Part model, mm, in its own coordinate system. Give positions to 0.01 mm unless a question says otherwise; leave off trailing zeros. Write each loop counter-clockwise with the first axis right and the second up, starting at its lowest first coordinate (ties: lowest second). Pieces come first, ordered by that corner, then holes. Notation, with made-up numbers: M 77.25,-19 L 116.25,-19 A20 ccw 116.25,20 Z; hole C 39,82.25 d2. An arc over 180 degrees is marked long. Answer as CSV lines item,"result". Start each with the question number.
1) Slice it at A-A, the plane y = -63.5. Give the cut face in (x, z), plus the area to 3 significant figures.
2) Pin check, flat tip, straight feed: pin 1 Ø15.5 at (x, y) = (-84, 0) entering from +Z. Stop position of the tip, or through.
3) Slice it at D-D, the plane z = 1.75. Give the number of separate pieces and of enclosed holes in the cut face, plus the area to 3 significant figures.
4) Slice it at B-B, the plane x = 28. Give the cut face in (y, z).
5) Wall check: line 1 along Y through (x, z) = (-28, 4); line 2 along X through (y, z) = (0, 6); line 3 along Y through (x, z) = (84, 2.75). Give the ranges that are in metal, low to high. Write a range as from..to.
6) Slice it at C-C, the plane y = -127. Give the cut face in (x, z).
Autodesk Inventor part; units mm, degrees
ref_plane "YZ Plane" through (0, 0, 0) normal (1, 0, 0) x (0, 1, 0)
ref_plane "XZ Plane" through (0, 0, 0) normal (0, 1, 0) x (-1, 0, 0)
ref_plane "XY Plane" through (0, 0, 0) normal (0, 0, 1) x (1, 0, 0)
sketch "Sketch2" plane through (0, 0, 0) normal (0, 0, 1) x (1, 0, 0)
  line L0 (-53, -96) -> (53, -96)
  line L1 (53, -96) -> (53, 96)
  line L2 (53, 96) -> (-53, 96)
  line L3 (-53, 96) -> (-53, -96)
  line L4 (-53, -96) -> (53, 96) construction
  line L5 (53, -96) -> (-53, 96) construction
  line L6 (-103, -146) -> (103, -146)
  line L7 (103, -146) -> (103, 146)
  line L8 (103, 146) -> (-103, 146)
  line L9 (-103, 146) -> (-103, -146)
  point P0 (0, 0)
  dimension "d29" = 106
  dimension "d30" = 192
  dimension "d31" = 50
extrude "Plate2" add sketch "Sketch2" along normal blind 8
sketch "Sketch5" plane through (0, 0, 8) normal (0, 0, 1) x (1, 0, 0)
  line L0 (53, 96) -> (53, -96) construction
  line L1 (53, -96) -> (-53, -96) construction
  line L2 (-53, -96) -> (-53, 96) construction
  line L3 (-53, 96) -> (53, 96) construction
  line L4 (103, -146) -> (-103, -146) construction
  line L5 (103, 146) -> (103, -146) construction
  line L6 (-103, 146) -> (103, 146) construction
  line L7 (-103, -146) -> (-103, 146) construction
  line L8 (-84, 127) -> (84, 127) construction
  line L9 (84, 127) -> (84, -127) construction
  line L10 (84, -127) -> (-84, -127) construction
  line L11 (-84, -127) -> (-84, 127) construction
  line L12 (-53, 0) -> (53, 0) construction
  line L13 (0, 96) -> (0, -96)
  point P0 (0, 0)
  point P1 (0, -127)
  point P2 (-84, 63.5)
  point P3 (-84, 0)
  point P4 (-84, -63.5)
  point P5 (-28, -127)
  point P6 (28, -127)
  point P7 (84, -63.5)
  point P8 (84, 0)
  point P9 (84, 63.5)
  point P10 (28, 127)
  point P11 (-28, 127)
  dimension "d34" = 19
  dimension "d49" = 63.5
  dimension "d50" = 63.5
  dimension "d51" = 56
  dimension "d52" = 56
  dimension "d53" = 56
fillet "Corner Round1" radius 6 8 edges at (-103, -146, 4) (-103, 146, 4) (103, 146, 4) (103, -146, 4) (53, -96, 4) (-53, -96, 4) (-53, 96, 4) (53, 96, 4)
hole "Hole1" at (-84, 127, 8) at (-84, 63.5, 8) at (-84, 0, 8) at (-84, -63.5, 8) at (-84, -127, 8) at (-28, -127, 8) at (28, -127, 8) at (84, -127, 8) at (84, -63.5, 8) at (84, 0, 8) at (84, 63.5, 8) at (84, 127, 8) at (28, 127, 8) at (-28, 127, 8) direction (0, 0, -1) diameter 17 end through all
equation "\"d29\" = ChargingHatch_hight - 2 * Thickness"
equation "\"d30\" = ChargingHatch_width - 2 * Thickness"
equation "\"d59\" = Thickness"
equation "\"d14\" = Thickness"
equation "\"BendReliefWidth\" = Thickness"
equation "\"BendReliefDepth\" = 0.5 * Thickness"
equation "\"CornerReliefSize\" = 4 * Thickness"
equation "\"MinimumRemnant\" = 2 * Thickness"
equation "\"TransitionRadius\" = BendRadius"
equation "\"JacobiRadiusSize\" = BendRadius"
equation "\"GapSize\" = Thickness"
properties part number "PRS 9606 charging flange round_D1200 940" material "Steel"
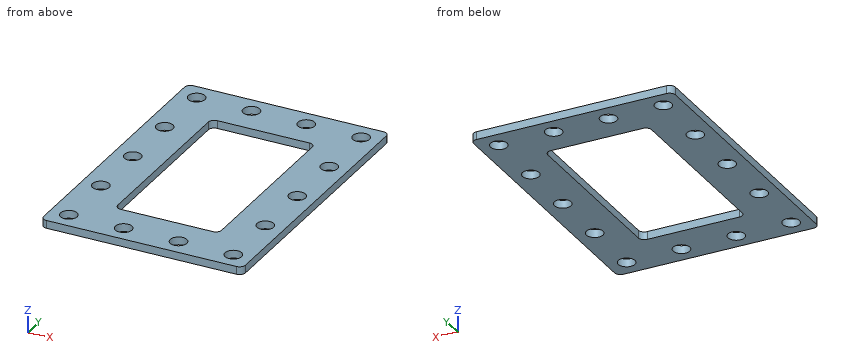
Found:
1,outline,"M -103,0 L -92.5,0 L -92.5,8 L -103,8 Z; M -75.5,0 L -53,0 L -53,8 L -75.5,8 Z; M 53,0 L 75.5,0 L 75.5,8 L 53,8 Z; M 92.5,0 L 103,0 L 103,8 L 92.5,8 Z"
1,area,"528 mm²"
2,pin 1,"through"
3,separate pieces,"1"
3,enclosed holes,"15"
3,area,"36,600 mm²"
4,outline,"M -146,0 L -135.5,0 L -135.5,8 L -146,8 Z; M -118.5,0 L -96,0 L -96,8 L -118.5,8 Z; M 96,0 L 118.5,0 L 118.5,8 L 96,8 Z; M 135.5,0 L 146,0 L 146,8 L 135.5,8 Z"
5,line 1,"-146..-135.5, -118.5..-96, 96..118.5, 135.5..146"
5,line 2,"-103..-92.5, -75.5..-53, 53..75.5, 92.5..103"
5,line 3,"-146..-135.5, -118.5..-72, -55..-8.5, 8.5..55, 72..118.5, 135.5..146"
6,outline,"M -103,0 L -92.5,0 L -92.5,8 L -103,8 Z; M -75.5,0 L -36.5,0 L -36.5,8 L -75.5,8 Z; M -19.5,0 L 19.5,0 L 19.5,8 L -19.5,8 Z; M 36.5,0 L 75.5,0 L 75.5,8 L 36.5,8 Z; M 92.5,0 L 103,0 L 103,8 L 92.5,8 Z"
